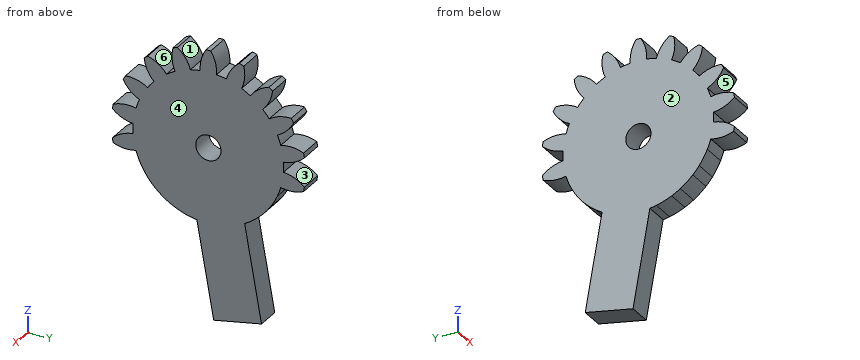
```python
from build123d import *

# Parameters (mm, degrees)
BASPROSKE_W                  = 3.175
BASPROSKE_H                  = 12.7
TOOTHCUT_DEPTH               = 19.238986403
TEETHCUTS_COUNT              = 18
TEETHCUTS_ANGLE              = 340
BORSKE_R                     = 1.5875
BORE_DEPTH                   = 50.8000508
CUT_EXTRUDE_THIN1_DEPTH      = 2.54
CUT_EXTRUDE_THIN1_DEPTH_BACK = 5.08
BOSS_EXTRUDE1_DEPTH          = 3.175
SKETCH9_R                    = 1.651
CUT_EXTRUDE2_DEPTH           = 3.175


with BuildPart() as part:
    # BasProSke → Base-Revolve (revolve)
    with BuildSketch(Plane(origin=(0, 0, 0), x_dir=(1, 0, 0), z_dir=(0, 1, 0)), mode=Mode.PRIVATE) as base_revolve_sk:
        with Locations((1.5875, 6.35)):
            Rectangle(BASPROSKE_W, BASPROSKE_H)
    revolve(base_revolve_sk.sketch.rotate(Axis((-10, 0, 0), (1, 0, 0)), 180), axis=Axis((-10, 0, 0), (1, 0, 0)))

    # TooCutSke → ToothCut (cut, through all)
    with BuildSketch(Plane(origin=(0, 0, 0), x_dir=(0, 0, -1), z_dir=(1, 0, 0))):
        with BuildLine():
            ThreePointArc((0.653663469, 9.833498417), (0, 9.8552), (-0.653663469, 9.833498417))
            ThreePointArc((-0.653663469, 9.833498417), (-1.05484238, 11.314407704), (-1.923354389, 12.579209556))
            ThreePointArc((-1.923354389, 12.579209556), (0, 12.7254), (1.923354389, 12.579209556))
            ThreePointArc((1.923354389, 12.579209556), (1.05484238, 11.314407704), (0.653663469, 9.833498417))
        make_face()
    toothcut = extrude(amount=TOOTHCUT_DEPTH, mode=Mode.SUBTRACT)

    # TeethCuts: ToothCut ×18 about axis
    teethcuts_axis = Axis((-10, 0, 0), (1, 0, 0))
    for i in range(1, TEETHCUTS_COUNT):
        add(toothcut.rotate(teethcuts_axis, i * TEETHCUTS_ANGLE / (TEETHCUTS_COUNT - 1)), mode=Mode.SUBTRACT)

    # BorSke → Bore (cut, symmetric)
    with BuildSketch(Plane(origin=(0, 0, 0), x_dir=(0, 0, -1), z_dir=(1, 0, 0))):
        with Locations(Location((0, 0, 0), (0, 0, 180))):
            Circle(BORSKE_R)
    extrude(amount=BORE_DEPTH, both=True, mode=Mode.SUBTRACT)

    # Sketch7 → Cut-Extrude-Thin1 (cut, two sides: drawn at the far end of the back side and taken through both)
    with BuildSketch(Plane.ZY.offset(-CUT_EXTRUDE_THIN1_DEPTH_BACK)):
        with BuildLine():
            Line((-10.823936545, 10.290898732), (-25.264431922, 12.837147681))
            Line((-25.264431922, 12.837147681), (-28.131363335, -3.422028321))
            Line((-28.131363335, -3.422028321), (-13.690867959, -5.968277271))
            ThreePointArc((-13.690867959, -5.968277271), (-11.782416361, -9.177955314), (-9.137407483, -11.813889433))
            Line((-9.137407483, -11.813889433), (-10.123749891, -15.359323522))
            ThreePointArc((-10.123749891, -15.359323522), (18.392184669, -0.355912967), (-9.521946872, 15.739493597))
            Line((-9.521946872, 15.739493597), (-8.708557038, 12.133475733))
            ThreePointArc((-8.708557038, 12.133475733), (-9.809604931, 11.261964755), (-10.823936545, 10.290898732))
        make_face()
        with BuildLine():
            Line((-8.636682816, 4.746859697), (-21.143741279, 6.952191553))
            Line((-21.143741279, 6.952191553), (-22.246407207, 0.698662322))
            Line((-22.246407207, 0.698662322), (-9.739348744, -1.506669535))
            ThreePointArc((-9.739348744, -1.506669535), (-7.549024322, -6.335392555), (-3.17353646, -9.330253661))
            Line((-3.17353646, -9.330253661), (-4.102105036, -12.668018169))
            ThreePointArc((-4.102105036, -12.668018169), (13.313553301, -0.235050135), (-3.652381497, 12.804923251))
            Line((-3.652381497, 12.804923251), (-2.889344669, 9.422136405))
            ThreePointArc((-2.889344669, 9.422136405), (-6.219073923, 7.64513483), (-8.636682816, 4.746859697))
        make_face(mode=Mode.SUBTRACT)
    extrude(amount=CUT_EXTRUDE_THIN1_DEPTH + CUT_EXTRUDE_THIN1_DEPTH_BACK, mode=Mode.SUBTRACT)

    # Sketch8 → Boss-Extrude1 (add)
    with BuildSketch(Plane.ZY):
        Polygon((-21.143741279, 6.952191553), (-22.246407207, 0.698662322), (-9.739348744, -1.506669535), (-8.636682816, 4.746859697), align=None)
    extrude(amount=-BOSS_EXTRUDE1_DEPTH)

    # Sketch9 → Cut-Extrude2 (cut)
    with BuildSketch(Plane.ZY):
        Circle(SKETCH9_R)
    extrude(amount=-CUT_EXTRUDE2_DEPTH, mode=Mode.SUBTRACT)


solid = part.part
```
The model under review builds one solid part; all positions refer to its coordinate system, in mm. Face numbers are marked on the shaded views. A direction names the side the tool comes from. Coordinates: 2 decimals unless noted, no trailing zeros. Write each loop counter-clockwise with the first axis right and the second up, starting at its lowest first coordinate (ties: lowest second). Pieces come first, ordered by that corner, then holes.
1) Clearance check with flat-ended pins moving along their axes: pin 1 Ø2.5 at (y, z) = (0, 0) entering from +X; pin 2 Ø1 at (x, z) = (2.5, -7.5) entering from +Y. State where each tip first meets the part, or that it passes through.
2) We need section C-C on z = -3.5. State the section outline as (x, y) points (3 decimals).
3) Machinability: for the marked faces 4, 5 and 6, which of the approach directions +Z, -Z, +X, -X, +Y, -Y give a long, thin tool a straight path to every point of the face, cutting with its end or side? Answer none if there is none.
4) We need section A-A on z = 0. State the section outline as (x, y) points (3 decimals), then the cut area to 3 significant figures.
5) We need section B-B on y = -6.5. State the section outline as (x, z) points (3 decimals).
6) The part is to be moulded in two halves that separate along Z. For the marked faces 1, 2 and 3, say which applies: pulls with the +Z half, pulls with the -Z half, needs draft (parallel to the pull), parting line crosses it, or undercut.
7) To check wall thickness, follow probe 1 along Y at (x, z) = (2.3, 0); probe 2 along Z at (x, y) = (1.8, 7.25); probe 3 along Z at (x, y) = (2.7, -8). State the ranges of each line that lie inside material, in increasing order.
Answer list:
1. pin 1: passes through
1. pin 2: stops at y = 6.94
2. outline: (0, -9.213) - (3.175, -9.213) - (3.175, 9.213) - (0, 9.213) - close
3. face 4: +Z, -Z, +X, +Y, -Y
3. face 5: +X, -X, -Y
3. face 6: +Z, +X, -X
4. outline: (0, -9.855) - (3.175, -9.855) - (3.175, -1.651) - (0, -1.651) - close; (0, 1.651) - (3.175, 1.651) - (3.175, 9.855) - (0, 9.855) - close
4. area: 52.1 mm2
5. outline: (0, -7.408) - (3.175, -7.408) - (3.175, 9.22) - (0, 9.22) - close
6. face 1: pulls with the +Z half
6. face 2: needs draft
6. face 3: undercut
7. probe 1: y = -9.86 to -1.65, 1.65 to 9.86
7. probe 2: z = -6.68 to 6.68, 6.97 to 9.67
7. probe 3: z = -5.76 to 5.85, 8.1 to 9.86
